from build123d import *

# Parameters (mm, degrees)
SKETCH003_R  = 5.5
PAD001_DEPTH = 51.4
PAD_DEPTH    = 56
SKETCH002_R  = 2.5
POCKET_DEPTH = 6
FILLET_R     = 3
SKETCH004_R  = 19.05
PAD002_DEPTH = 1.6
SKETCH005_R  = 3.175
PAD003_DEPTH = 19
FILLET001_R  = 0.5


with BuildPart() as pad001:
    # Sketch003 → Pad001 (new body)
    with BuildSketch(Plane.XY.offset(-1)):
        with Locations((-23.55, 23.55)):
            Circle(SKETCH003_R)
        with Locations((-23.55, -23.55)):
            Circle(SKETCH003_R)
        with Locations((23.55, 23.55)):
            Circle(SKETCH003_R)
        with Locations((23.55, -23.55)):
            Circle(SKETCH003_R)
    extrude(amount=PAD001_DEPTH)


with BuildPart() as fillet001:
    # Sketch → Pad (new body)
    with BuildSketch(Plane.XY):
        with BuildLine():
            Line((-25.2, 28.2), (25.2, 28.2))
            ThreePointArc((28.2, 25.2), (27.32132, 27.32132), (25.2, 28.2))
            Line((28.2, 25.2), (28.2, -25.2))
            ThreePointArc((25.2, -28.2), (27.32132, -27.32132), (28.2, -25.2))
            Line((25.2, -28.2), (-25.2, -28.2))
            ThreePointArc((-28.2, -25.2), (-27.32132, -27.32132), (-25.2, -28.2))
            Line((-28.2, -25.2), (-28.2, 25.2))
            ThreePointArc((-25.2, 28.2), (-27.32132, 27.32132), (-28.2, 25.2))
        make_face()
    extrude(amount=PAD_DEPTH)

    # Sketch002 → Pocket (cut)
    with BuildSketch(Plane.XY.offset(56)):
        with Locations((-23.55, 23.55)):
            Circle(SKETCH002_R)
        with Locations((-23.55, -23.55)):
            Circle(SKETCH002_R)
        with Locations((23.55, 23.55)):
            Circle(SKETCH002_R)
        with Locations((23.55, -23.55)):
            Circle(SKETCH002_R)
    extrude(amount=-POCKET_DEPTH, mode=Mode.SUBTRACT)

    # Cut: cut Pad001
    add(pad001.part, mode=Mode.SUBTRACT)

    # Fillet
    fillet_edges = [fillet001.edges().sort_by_distance(p)[0] for p in [
        (-20.612739, -28.2, 25.2),
        (-28.2, -20.612739, 25.2),
        (-28.2, 20.612739, 25.2),
        (-20.612739, 28.2, 25.2),
        (20.612739, 28.2, 25.2),
        (28.2, 20.612739, 25.2),
        (28.2, -20.612739, 25.2),
        (20.612739, -28.2, 25.2),
    ]]
    fillet(fillet_edges, radius=FILLET_R)

    # Sketch004 → Pad002 (new body)
    with BuildSketch(Plane.XY.offset(56)):
        with Locations((0.021046, -0.026368)):
            Circle(SKETCH004_R)
    extrude(amount=PAD002_DEPTH)

    # Sketch005 → Pad003 (new body)
    with BuildSketch(Plane.XY.offset(57.6)):
        with Locations((-0.017815, 0.022992)):
            Circle(SKETCH005_R)
    extrude(amount=PAD003_DEPTH)

    # Fillet001
    fillet001_edges = [fillet001.edges().sort_by_distance(p)[0] for p in [
        (-3.192815, 0.022992, 76.6),
    ]]
    fillet(fillet001_edges, radius=FILLET001_R)


solid = fillet001.part
The listing builds one solid part. Answer for the finished solid, in the listing's coordinates (mm). A direction names the side the tool comes from. Round coordinates to 2 decimals unless told otherwise and drop trailing zeros. Order: outer loops, then holes, each group sorted by start corner. A loop starts at its lowest first (then second) coordinate and runs counter-clockwise, first axis right, second up. Notation, with made-up numbers: (34.25, -8) -> (46.25, -8) arc R15 cw to (46.25, 17) -> close; hole circle Ø4 at (7, 80.5). An arc over 180 degrees is marked (long way). One line per item, written item: value.
Item 1: Straight lines are drawn through the part: L1, parallel to Y at x = -23.55, z = 54.95; L2, parallel to X at y = -23, z = 52; L3, parallel to Y at x = -25, z = 6. For each, find the intervals that lie inside material, in ascending order.
Taken from the geometry:
L1: y = -28.2 to -26.05, -21.05 to 21.05, 26.05 to 28.2
L2: x = -28.2 to -25.99, -21.11 to 21.11, 25.99 to 28.2
L3: y = -18.21 to 18.21
Item 2: Find section D-D, the plane z = 10. Give the vertices of the cut face in (x, y).
Taken from the geometry:
outline: (-28.2, -15.21) arc R3 ccw to (-24.62, -18.15) arc R5.5 cw to (-18.15, -24.62) arc R3 ccw to (-15.21, -28.2) -> (15.21, -28.2) arc R3 ccw to (18.15, -24.62) arc R5.5 cw to (24.62, -18.15) arc R3 ccw to (28.2, -15.21) -> (28.2, 15.21) arc R3 ccw to (24.62, 18.15) arc R5.5 cw to (18.15, 24.62) arc R3 ccw to (15.21, 28.2) -> (-15.21, 28.2) arc R3 ccw to (-18.15, 24.62) arc R5.5 cw to (-24.62, 18.15) arc R3 ccw to (-28.2, 15.21) -> close
Item 3: For faces 5 (the flat face through (-28.2, 0, 28)), 6 (the cylindrical face through (18.19, 5.7, 56.79)), determine the directions among +Z, -Z, +X, -X, +Y, -Y from which every point of the face is accessible in a straight line to the end or side of a thin tool.
Taken from the geometry:
face 5: +Z, -Z, -X, +Y, -Y
face 6: +Z
Item 4: Find section A-A, the plane x = -23.55. Give the vertices of the cut face in (y, z), then the cut area to 3 significant figures.
Taken from the geometry:
outline: (-28.2, 50.4) -> (-26.05, 50.4) -> (-26.05, 56) -> (-28.2, 56) -> close; (-21.05, 50.4) -> (-18.05, 50.4) -> (-18.05, 0) -> (18.05, 0) -> (18.05, 50.4) -> (21.05, 50.4) -> (21.05, 56) -> (-21.05, 56) -> close; (26.05, 50.4) -> (28.2, 50.4) -> (28.2, 56) -> (26.05, 56) -> close
area: 2,080 mm2
Item 5: Given P1, Ø4, axis at x = -24.5, y = 24, coming from the -Z side; P2, Ø8, axis at x = -23.55, y = 23.55, coming from the +Z side; P3, Ø6, axis at x = -5, y = -9, coming from the +Z side, each flat-ended and moving along its own axis, determine where each tip first touches the part or whether it passes through.
Taken from the geometry:
P1: stops at z = 50.4
P2: stops at z = 56
P3: stops at z = 57.6
Item 6: Find section C-C, the plane x = 17. Give the vertices of the cut face in (y, z), then the cut area to 3 significant figures.
Taken from the geometry:
outline: (-28.2, 50.4) -> (-27.61, 50.4) -> (-27.61, 0) -> (27.61, 0) -> (27.61, 50.4) -> (28.2, 50.4) -> (28.2, 56) -> (8.61, 56) -> (8.61, 57.6) -> (-8.66, 57.6) -> (-8.66, 56) -> (-28.2, 56) -> close
area: 3,130 mm2
Item 7: For a pull along Y with two mould halves and no side action, classify faces 1 (the flat face through (28.2, 0, 28)), 2 (the cylindrical face through (19.71, -19.61, 24.85)), 3 (the flat face through (0, 28.2, 28)), 4 (the cylindrical face through (-19.71, 19.61, 24.85)) as released by +Y, released by -Y, zero draft, split by the parting line, or undercut.
Taken from the geometry:
face 1: zero draft
face 2: undercut
face 3: released by +Y
face 4: undercut
